from build123d import *

# Parameters (mm, degrees)
F2_W     = 0.5
F2_H     = 2
F2_W_2   = 1
F3_DEPTH = 2


with BuildPart() as f3:
    # F2 (on offset) → F3 (new body)
    with BuildSketch(Plane.XY.offset(10)):
        with Locations((-0.25, 1.5)):
            Rectangle(F2_W, F2_H)
        with Locations((0.25, 1.5)):
            Rectangle(F2_W, F2_H)
        Polygon((0.5, 0.5), (0, 0.5), (-0.5, 0.5), (-0.5, 0), (-0.5, -0.5), (0.5, -0.5), (0.5, 0), align=None)
        Polygon((2.5, 0.5), (0.5, 0.5), (0.5, 0), (0.5, -0.5), (2.5, -0.5), align=None)
        Polygon((-0.5, 0), (-0.5, 0.5), (-2.5, 0.5), (-2.5, -0.5), (-0.5, -0.5), align=None)
        with Locations((0, -1.5)):
            Rectangle(F2_W_2, F2_H)
    extrude(amount=-F3_DEPTH)

    # F0 (on Front) → F4 (revolve)
    with BuildSketch(Plane.XZ):
        with BuildLine():
            ThreePointArc((2.5, 30), (1.563711, 25.038911), (1.25, 20))
            Line((1.25, 20), (2.25, 20))
            ThreePointArc((2.25, 20), (2.563711, 25.038911), (3.5, 30))
            Line((3.5, 30), (3.5, 40))
            Line((3.5, 40), (2.5, 40))
            Line((2.5, 40), (2.5, 30))
        make_face()
        with BuildLine():
            Line((2.5, 10), (2.5, 0))
            Line((2.5, 0), (3.5, 0))
            Line((3.5, 0), (3.5, 10))
            ThreePointArc((3.5, 10), (2.563711, 14.961089), (2.25, 20))
            Line((2.25, 20), (1.25, 20))
            ThreePointArc((1.25, 20), (1.563711, 14.961089), (2.5, 10))
        make_face()
    revolve(axis=Axis((0, 0, 20), (0, 0, 1)))


solid = f3.part
Build history of the part. All positions in model axes, mm. A direction names the side the tool comes from. Give positions to 0.01 mm unless a question says otherwise; leave off trailing zeros. Loops run counter-clockwise (first coordinate to the right, second up) from the corner with the lowest first, then second, coordinate; pieces in that order, holes last. Notation, with made-up numbers: (6.25, 68.5) -> (21.25, 68.5) arc R19 ccw to (21.25, 85.5) -> close; hole circle Ø11 at (-33.75, -33). An arc over 180 degrees is marked (long way). Answer in a Markdown table with one row per item.
Item 1: Mould opens along X. For faces 4 (the flat face through (0.5, -1, 9)), 5 (the cylindrical face through (3.233, -1.341, 35.07)), 6 (the flat face through (2, -2, 40)) say: pulls with the +X half, pulls with the -X half, needs draft (parallel to the pull), parting line crosses it, or undercut.
Findings below:
| item | result |
|---|---|
| face 4 | undercut |
| face 5 | parting line crosses it |
| face 6 | needs draft |
Item 2: Tool access for faces 1 (the cylindrical face through (-0.54, -2.44, 34.93)), 2 (the flat face through (1, 0.5, 9)), 3 (the flat face through (0, 0, 10)): list every direction of +Z, -Z, +X, -X, +Y, -Y with a clear straight run to the whole face (end or side of a thin tool).
Findings below:
| item | result |
|---|---|
| face 1 | +Z |
| face 2 | -Z |
| face 3 | none |
Item 3: Slice it at B-B on y = 0. Write the cut outline in (x, z).
Findings below:
| item | result |
|---|---|
| outline | (-3.5, 0) -> (-2.5, 0) -> (-2.5, 8) -> (2.5, 8) -> (2.5, 0) -> (3.5, 0) -> (3.5, 10) arc R40.62 cw to (2.25, 20) arc R40.62 cw to (3.5, 30) -> (3.5, 40) -> (2.5, 40) -> (2.5, 30) arc R40.62 ccw to (1.25, 20) arc R40.62 ccw to (2.5, 10) -> (-2.5, 10) arc R40.62 ccw to (-1.25, 20) arc R40.62 ccw to (-2.5, 30) -> (-2.5, 40) -> (-3.5, 40) -> (-3.5, 30) arc R40.62 cw to (-2.25, 20) arc R40.62 cw to (-3.5, 10) -> close |
Item 4: Flat gauge pins, fed straight in: P1, Ø4, axis at x = -0.5, y = 1, coming from the +Z side; P2, Ø2, axis at x = 2, z = 8.5, coming from the +Y side; P3, Ø1, axis at y = 1, z = 9.5, coming from the +X side; P4, Ø2, axis at x = 1.5, z = 9, coming from the -Y side. Where does each tip first touch, or does it go through?
Findings below:
| item | result |
|---|---|
| P1 | stops at z = 40 |
| P2 | stops at y = 3.35 |
| P3 | stops at x = 3.46 |
| P4 | stops at y = -3.46 |
Item 5: Slice it at A-A on z = 9. Write the cut outline in (x, y).
Findings below:
| item | result |
|---|---|
| outline | circle Ø7 at (0, 0); hole (-2.45, -0.5) arc R2.5 ccw to (-0.5, -2.45) -> (-0.5, -0.5) -> close; hole (-2.45, 0.5) -> (-0.5, 0.5) -> (-0.5, 2.45) arc R2.5 ccw to start; hole (0.5, -2.45) arc R2.5 ccw to (2.45, -0.5) -> (0.5, -0.5) -> close; hole (0.5, 0.5) -> (2.45, 0.5) arc R2.5 ccw to (0.5, 2.45) -> close |
Item 6: Slice it at D-D on z = 5. Write the cut outline in (x, y), plus the area to 3 significant figures.
Findings below:
| item | result |
|---|---|
| outline | circle Ø7 at (0, 0); hole circle Ø5 at (0, 0) |
| area | 18.8 mm² |
Item 7: Probe line 1 along Y through (x, z) = (0, 34); line 2 along X through (y, z) = (0.5, 34); line 3 along X through (y, z) = (0.25, 26). List the from-to ranges inside material, lowest first. Write a range as [from, to].
Findings below:
| item | result |
|---|---|
| line 1 | y = [-3.5, -2.5], [2.5, 3.5] |
| line 2 | x = [-3.46, -2.45], [2.45, 3.46] |
| line 3 | x = [-2.68, -1.68], [1.68, 2.68] |
